Read the model definition and answer for the solid it produces. Units are mm, in the model's axes. Give positions to 0.01 mm unless a question says otherwise; leave off trailing zeros. Write each loop counter-clockwise with the first axis right and the second up, starting at its lowest first coordinate (ties: lowest second). Pieces come first, ordered by that corner, then holes. Notation, with made-up numbers: M 64.5,-30.5 L 112.5,-30.5 A26 cw 112.5,2.5 Z; hole C 6,23 d8. An arc over 180 degrees is marked long. Put each result on its own line as item: value.
from build123d import *

# Parameters (mm, degrees)
F0_W     = 50.8
F0_H     = 6.731
F0_R     = 2.3114
F1_DEPTH = 10.16
F3_W     = 50.8
F3_H     = 10.16
F4_DEPTH = 10.16
F5_R     = 2.3114
F6_DEPTH = 70.36535
F7_R     = 5.08


with BuildPart() as f1:
    # F0 (on Top) → F1 (new body)
    with BuildSketch(Plane.XY):
        Rectangle(F0_W, F0_H)
        with Locations((-7.62, 0)):
            Circle(F0_R, mode=Mode.SUBTRACT)
        with Locations((7.62, 0)):
            Circle(F0_R, mode=Mode.SUBTRACT)
    extrude(amount=F1_DEPTH)

    # F3 (on face) → F4 (join)
    with BuildSketch(Plane.XZ.offset(3.3655)):
        with Locations((0, 5.08)):
            Rectangle(F3_W, F3_H)
    extrude(amount=F4_DEPTH)

    # F5 (on face) → F6 (cut)
    with BuildSketch(Plane.YZ.offset(25.4)):
        with Locations((-9.919893, 4.456782)):
            Circle(F5_R)
    extrude(amount=-F6_DEPTH, mode=Mode.SUBTRACT)

    # F7
    f7_edges = [f1.edges().sort_by_distance(p)[0] for p in [
        (-25.4, 3.3655, 5.08),
        (25.4, 3.3655, 5.08),
    ]]
    fillet(f7_edges, radius=F7_R)


solid = f1.part
(1) Section B-B on z = 9.5 is taken. Determine the outline of the cut face in (x, y), and give its area (3 significant figures).
Result:
outline: M -25.4,-13.53 L 25.4,-13.53 L 25.4,-1.71 A5.08 ccw 20.32,3.37 L -20.32,3.37 A5.08 ccw -25.4,-1.71 Z; hole C -7.62,0 d4.62; hole C 7.62,0 d4.62
area: 813 mm²
(2) Straight lines are drawn through the part: line 1 along Y through (x, z) = (7.5, 5.75); line 2 along Y through (x, z) = (-7.62, 3.5); line 3 along Y through (x, z) = (19, 4.5). For each, find the intervals that lie inside material, in ascending order. Write a range as from..to.
Result:
line 1: y = -13.53..-11.84, -8..-2.31, 2.31..3.37
line 2: y = -13.53..-12.02, -7.82..-2.31, 2.31..3.37
line 3: y = -13.53..-12.23, -7.61..3.37
(3) Section A-A on x = -7.62 is taken. Determine the outline of the cut face in (y, z).
Result:
outline: M -13.53,0 L -2.31,0 L -2.31,10.16 L -13.53,10.16 Z; M 2.31,0 L 3.37,0 L 3.37,10.16 L 2.31,10.16 Z; hole C -9.92,4.46 d4.62
(4) For a pull along X with two mould halves and no side action, classify faces 1 (the face through (9.755, -0.885, 5.009)), 2 (the face through (-23.95, 1.84, 5.15)), 3 (the face through (0, -5, 10.16)) as +X half, -X half, draft (parallel to the pull), parting line (faces both ways), or undercut.
Result:
face 1: undercut
face 2: -X half
face 3: draft
(5) Given pin 1 Ø1 at (y, z) = (-1, 2.5) entering from +X, flat-ended and moving along its own axis, determine where the tip first touches the part or whether it passes through.
Result:
pin 1: stops at x = 25.4
(6) Section C-C on y = 0 is taken. Determine the outline of the cut face in (x, z), and give its area (3 significant figures).
Result:
outline: M -25.1,0 L -9.93,0 L -9.93,10.16 L -25.1,10.16 Z; M -5.31,0 L 5.31,0 L 5.31,10.16 L -5.31,10.16 Z; M 9.93,0 L 25.1,0 L 25.1,10.16 L 9.93,10.16 Z
area: 416 mm²
